Input: part model. Units: mm. Frame: model coordinates. A direction names the side the tool comes from. Give positions to 0.01 mm unless a question says otherwise; leave off trailing zeros. Loops run counter-clockwise (first coordinate to the right, second up) from the corner with the lowest first, then second, coordinate; pieces in that order, holes last. Notation, with made-up numbers: (58.25, 35) - (108.25, 35) arc R21 cw to (108.25, 44) - close; hole circle Ø5 at (-3.5, 12.25). An arc over 180 degrees is marked (long way). One line per item, written item: value.
from build123d import *

# Parameters (mm, degrees)
SKETCH1_R             = 0.4
BOSS_EXTRUDE1_DEPTH   = 2
BOSS_EXTRUDE1_2_DEPTH = 2
SKETCH2_R             = 0.4
REVOLVE4_ANGLE        = 80
SKETCH3_R             = 0.4
REVOLVE5_ANGLE        = 30
SKETCH4_R             = 0.4
REVOLVE6_ANGLE        = 30
SKETCH11_R            = 0.4
SKETCH12_R            = 2.25
BOSS_EXTRUDE2_DEPTH   = 1.25
SKETCH13_R            = 0.4
REVOLVE7_ANGLE        = 30
SKETCH14_R            = 0.4
BOSS_EXTRUDE3_DEPTH   = 2


with BuildPart() as part:
    # Sketch1 → Boss-Extrude1 (new body)
    with BuildSketch(Plane(origin=(0, 0, 0), x_dir=(1, 0, 0), z_dir=(0, 1, 0))):
        with Locations(Location((-6.1, 0, 0), (0, 0, 270))):
            Circle(SKETCH1_R)
    extrude(amount=-BOSS_EXTRUDE1_DEPTH)



with BuildPart() as body_2:
    # Sketch1 → Boss-Extrude1 2 (new body)
    with BuildSketch(Plane(origin=(0, 0, 0), x_dir=(1, 0, 0), z_dir=(0, 1, 0))):
        with Locations(Location((6.1, 0, 0), (0, 0, 270))):
            Circle(SKETCH1_R)
    extrude(amount=-BOSS_EXTRUDE1_2_DEPTH)


with BuildPart() as part_1:
    add(part.part)

    add(body_2.part)  # Revolve4 merges body 2
    # Sketch2 → Revolve4 (revolve)
    with BuildSketch(Plane(origin=(0, 0, 0), x_dir=(1, 0, 0), z_dir=(0, 1, 0))):
        with Locations(Location((6.1, 0, 0), (0, 0, 270))):
            Circle(SKETCH2_R)
        with Locations(Location((-6.1, 0, 0), (0, 0, 270))):
            Circle(SKETCH2_R)
    revolve(axis=Axis((-6.5, 0, -0.5), (-1, 0, 0)), revolution_arc=REVOLVE4_ANGLE)

    # Sketch3 → Revolve5 (revolve)
    with BuildSketch(Plane(origin=(0, 0.085505036, -0.484923155), x_dir=(-1, 0, 0), z_dir=(0, 0.17364817766692736, -0.9848077530122086))):
        with Locations((-6.1, 0.413175911)):
            Circle(SKETCH3_R)
    revolve(axis=Axis((5.6, 0.982265488, -0.326800092), (0, 0.9848077530122086, 0.1736481776669274)), revolution_arc=REVOLVE5_ANGLE)

    # Sketch4 → Revolve6 (revolve)
    with BuildSketch(Plane(origin=(0, 0.085505036, -0.484923155), x_dir=(-1, 0, 0), z_dir=(0, 0.17364817766692736, -0.9848077530122086))):
        with Locations((6.1, 0.413175911)):
            Circle(SKETCH4_R)
    revolve(axis=Axis((-5.6, 1.037409724, -0.317076676), (0, -0.9848077530122086, -0.17364817766692733)), revolution_arc=REVOLVE6_ANGLE)

    # Sweep1: sweep along a path in Sketch5
    with BuildLine(Plane(origin=(0, 0.406898841, 0.071747244), x_dir=(1, 0, 0), z_dir=(0, 0.984807753012208, 0.17364817766693072))) as sweep1_path:
        ThreePointArc((-6.033012702, 0.742403877), (0, 4.225565384), (6.033012702, 0.742403877))
    # Sketch11 → Sweep1 (sweep)
    with BuildSketch(Plane(origin=(-1.186782867, -0.356945676, 2.024339523), x_dir=(-0.8402936458397423, -0.15403461860121453, -0.5197883463812287), z_dir=(0.5000000000000008, 0.15038373318043258, -0.8528685319524433))):
        with Locations((5.32970496, 1.754864912)):
            Circle(SKETCH11_R)
    sweep(path=sweep1_path.line)

    # Sketch12 → Boss-Extrude2 (add)
    with BuildSketch(Plane(origin=(0, 0.406898841, 0.071747244), x_dir=(1, 0, 0), z_dir=(0, 0.984807753012208, 0.17364817766693072))):
        with Locations(Location((0, 4.225565384, 0), (0, 0, 178.774322398))):
            Circle(SKETCH12_R)
    extrude(amount=BOSS_EXTRUDE2_DEPTH)

    # Sketch13 → Revolve7 (revolve)
    with BuildSketch(Plane.XZ.offset(2)):
        with Locations(Location((6.1, 0, 0), (0, 0, 90))):
            Circle(SKETCH13_R)
    revolve7 = revolve(axis=Axis((6.6, -2, -0.291841751), (0, 0, 1)), revolution_arc=REVOLVE7_ANGLE)

    # Sketch14 → Boss-Extrude3 (add)
    with BuildSketch(Plane(origin=(2.516025404, -4.357883832, 0), x_dir=(0.866025403784438, 0.500000000000001, 0), z_dir=(0.500000000000001, -0.866025403784438, 0))):
        with Locations(Location((4.215767665, 0, 0), (0, 0, 180))):
            Circle(SKETCH14_R)
    boss_extrude3 = extrude(amount=BOSS_EXTRUDE3_DEPTH)

    # Mirror1: Revolve7, Boss-Extrude3 across plane
    add(revolve7.mirror(Plane(origin=(0, 0, 0), x_dir=(0, 0, 1), z_dir=(1, 0, 0))))
    add(boss_extrude3.mirror(Plane(origin=(0, 0, 0), x_dir=(0, 0, 1), z_dir=(1, 0, 0))))


solid = part_1.part
Item 1: Section A-A, the plane y = -0.5. Output: boundary loops of the cut face in (x, z), and give its area (3 significant figures).
Verdict:
outline: circle Ø0.8 at (-6.1, 0); circle Ø0.8 at (6.1, 0)
area: 1.01 mm^2
Item 2: Draft query along Z for faces 3 (the face through (0.02, 0.91, -2.77)), 4 (the face through (0.054, 1.333, -5.181)), 5 (the face through (-5.703, -0.986, -0.052)). Return one class per face: pulls with the +Z half, pulls with the -Z half, needs draft (parallel to the pull), parting line crosses it, or undercut.
Verdict:
face 3: undercut
face 4: pulls with the -Z half
face 5: parting line crosses it
Item 3: Access query for faces 1 (the face through (0.031, 2.366, -3.841)), 2 (the face through (5.71, -0.99, -0.09)). Directions: +Z, -Z, +X, -X, +Y, -Y. A direction counts if a zero-diameter tool reaches every point of the face in a straight line with its end or side. Return the directions, or none.
Verdict:
face 1: +Z, +X, -X, +Y
face 2: none
Item 4: Material intervals for L1, parallel to X at y = -2.5, z = -0.25; L2, parallel to X at y = -1.5, z = -0.25; L3, parallel to Y at x = 6.5, z = 0.25, sorted ascending.
Verdict:
L1: x = -6.67 to -5.95, 5.95 to 6.67
L2: x = -6.41 to -5.79, 5.79 to 6.41
L3: y = -3.45 to -2.2
Item 5: Pin query (flat end, axial travel): P1, Ø1, axis at x = 1.5, z = -2, coming from the +Y side. Return the tip coordinate at first contact, or that it passes through.
Verdict:
P1: stops at y = 2.13
